from build123d import *

# Parameters (mm, degrees)
SKETCH1_R           = 3.5
BOSS_EXTRUDE1_DEPTH = 3


with BuildPart() as part:
    # Sketch1 → Boss-Extrude1 (new body)
    with BuildSketch(Plane(origin=(0, 0, 0), x_dir=(1, 0, 0), z_dir=(0, 1, 0))):
        Polygon((-54.142135624, 40), (-40, 54.142135624), (40, 54.142135624), (54.142135624, 40), (54.142135624, -40), (40, -54.142135624), (-40, -54.142135624), (-54.142135624, -40), align=None)
        with Locations((-21.213203436, 21.213203436)):
            Circle(SKETCH1_R, mode=Mode.SUBTRACT)
        with Locations((21.213203436, 21.213203436)):
            Circle(SKETCH1_R, mode=Mode.SUBTRACT)
        with Locations((21.213203436, -21.213203436)):
            Circle(SKETCH1_R, mode=Mode.SUBTRACT)
        with Locations((-21.213203436, -21.213203436)):
            Circle(SKETCH1_R, mode=Mode.SUBTRACT)
    extrude(amount=BOSS_EXTRUDE1_DEPTH)


solid = part.part
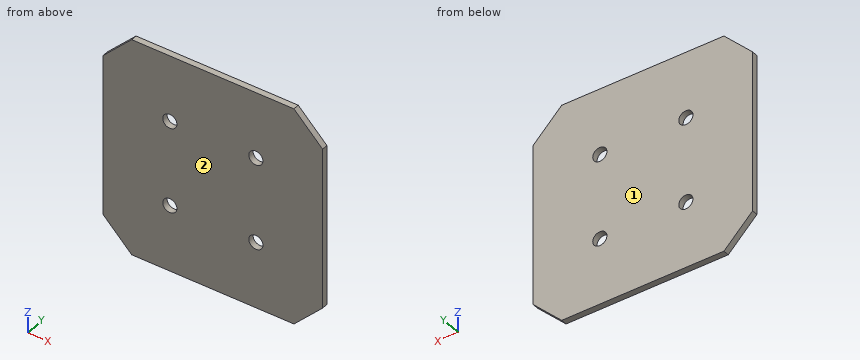
Work out the finished part from the listing and answer in its coordinate system (mm). Face numbers are marked on the shaded views. Give positions to 0.01 mm unless a question says otherwise; leave off trailing zeros. Loops run counter-clockwise (first coordinate to the right, second up) from the corner with the lowest first, then second, coordinate; pieces in that order, holes last. Notation, with made-up numbers: (-37.75, 23.25) - (-15.75, 23.25) arc R11 cw to (-15.75, 30.25) - close; hole circle Ø11 at (-23.75, 3). An arc over 180 degrees is marked (long way). Answer in a Markdown table with one row per item. Add a question column.
Q1. Each of these flat-tipped pins is pushed along its axis until it touches: P1, Ø3, axis at x = 17, z = -5, coming from the -Y side; P2, Ø6.5, axis at x = -21.21, z = 21.21, coming from the +Y side. Where does it stop, or does it pass through?
Q2. The part is cut by section B-B (x = 46). Determine the outline of the cut face in (y, z).
Q3. The part is cut by section A-A (y = 2.4). Determine the outline of the cut face in (x, z).
Q4. Determine the mould class of the marked faces 1 and 2 for opening direction Y: released by +Y, released by -Y, zero draft, split by the parting line, or undercut.
Q5. The part is cut by section C-C (z = -42.5). Determine the outline of the cut face in (x, y), and give its area (3 significant figures).
Q6. Consider line 1 along Z through (x, y) = (-21, 1.8); line 2 along X through (y, z) = (1.6, -21.5); line 3 along X through (y, z) = (0.7, -22). Determine where each line is inside the solid, lowest interval first.
Solution:
| question | item | result |
|---|---|---|
| 1 | P1 | stops at y = 0 |
| 1 | P2 | passes through |
| 2 | outline | (0, -48.14) - (3, -48.14) - (3, 48.14) - (0, 48.14) - close |
| 3 | outline | (-54.14, -40) - (-40, -54.14) - (40, -54.14) - (54.14, -40) - (54.14, 40) - (40, 54.14) - (-40, 54.14) - (-54.14, 40) - close; hole circle Ø7 at (-21.21, -21.21); hole circle Ø7 at (-21.21, 21.21); hole circle Ø7 at (21.21, -21.21); hole circle Ø7 at (21.21, 21.21) |
| 4 | face 1 | released by +Y |
| 4 | face 2 | released by -Y |
| 5 | outline | (-51.64, 0) - (51.64, 0) - (51.64, 3) - (-51.64, 3) - close |
| 5 | area | 310 mm² |
| 6 | line 1 | z = -54.14 to -24.71, -17.72 to 17.72, 24.71 to 54.14 |
| 6 | line 2 | x = -54.14 to -24.7, -17.72 to 17.72, 24.7 to 54.14 |
| 6 | line 3 | x = -54.14 to -24.62, -17.8 to 17.8, 24.62 to 54.14 |
